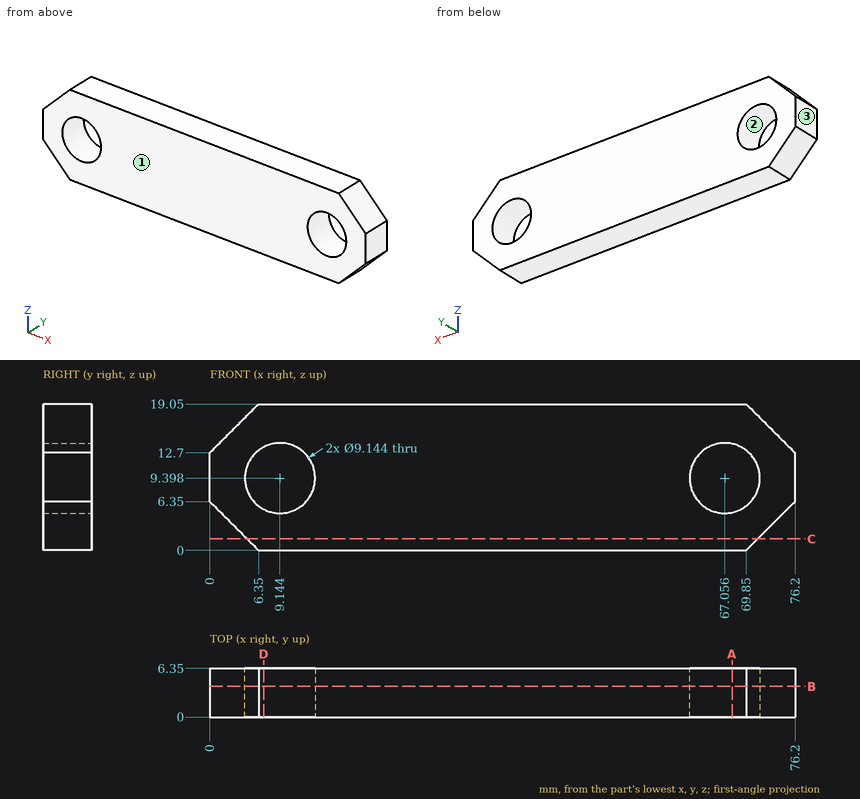
Input: dimensioned drawing with shaded views. Units: mm. Origin: part minimum x, y, z. Give positions to 0.01 mm unless a question says otherwise; leave off trailing zeros. Write each loop counter-clockwise with the first axis right and the second up, starting at its lowest first coordinate (ties: lowest second). Pieces come first, ordered by that corner, then holes.
1. Section query D-D (x = 7). Return the cut outline in (y, z), then the cut area to 3 significant figures.
2. Section query C-C (z = 1.5). Return the cut outline in (x, y), then the cut area to 3 significant figures.
3. Material intervals for line 1 along X through (y, z) = (1.25, 9.5); line 2 along X through (y, z) = (4.25, 7.25); line 3 along Z through (x, y) = (71, 3.5), sorted ascending.
4. Section query B-B (y = 4). Return the cut outline in (x, z), then the cut area to 3 significant figures.
5. Section query A-A (x = 68). Return the cut outline in (y, z).
6. Pull-direction query (X, two-part tool) for the marked faces 1, 2 and 3; classes: +X half, -X half, draft (parallel to the pull), parting line (faces both ways), or undercut.
7. First-contact query: pin 1 (7.5 mm diameter, centred on x = 67.056, z = 9.398, fed in from +Y). Flat tip, straight axial feed; report the tip coordinate or a pass-through.
Output values:
1. outline: (0, 0) - (6.35, 0) - (6.35, 5.36) - (0, 5.36) - close; (0, 13.44) - (6.35, 13.44) - (6.35, 19.05) - (0, 19.05) - close
1. area: 69.7 mm2
2. outline: (4.85, 0) - (71.35, 0) - (71.35, 6.35) - (4.85, 6.35) - close
2. area: 422 mm2
3. line 1: x = 0 to 4.57, 13.71 to 62.49, 71.63 to 76.2
3. line 2: x = 0 to 5.11, 13.18 to 63.02, 71.09 to 76.2
3. line 3: z = 1.15 to 7.09, 11.71 to 17.9
4. outline: (0, 6.35) - (6.35, 0) - (69.85, 0) - (76.2, 6.35) - (76.2, 12.7) - (69.85, 19.05) - (6.35, 19.05) - (0, 12.7) - close; hole circle Ø9.14 at (9.14, 9.4); hole circle Ø9.14 at (67.06, 9.4)
4. area: 1,240 mm2
5. outline: (0, 0) - (6.35, 0) - (6.35, 4.92) - (0, 4.92) - close; (0, 13.87) - (6.35, 13.87) - (6.35, 19.05) - (0, 19.05) - close
6. face 1: draft
6. face 2: undercut
6. face 3: -X half
7. pin 1: passes through
